Read the model definition and answer for the solid it produces. Units are mm, in the model's axes. Coordinates: 2 decimals unless noted, no trailing zeros. Order: outer loops, then holes, each group sorted by start corner. A loop starts at its lowest first (then second) coordinate and runs counter-clockwise, first axis right, second up. Notation, with made-up numbers: (42.5, 78) - (88.5, 78) arc R18 ccw to (88.5, 110) - close; hole circle Ø10 at (85, -21). An arc over 180 degrees is marked (long way). Use one line per item in the form item = value.
Autodesk Inventor part; units mm, degrees
ref_plane "YZ Plane" through (0, 0, 0) normal (1, 0, 0) x (0, 1, 0)
ref_plane "XZ Plane" through (0, 0, 0) normal (0, 1, 0) x (-1, 0, 0)
ref_plane "XY Plane" through (0, 0, 0) normal (0, 0, 1) x (1, 0, 0)
sketch "Sketch1" plane through (0, 0, 0) normal (0, 0, 1) x (1, 0, 0)
  line L0 (0, 0) -> (457.2, 0)
  line L1 (457.2, 0) -> (457.2, 304.8)
  line L2 (457.2, 304.8) -> (0, 304.8)
  line L3 (0, 304.8) -> (0, 0)
  line L4 (0, 254) -> (457.2, 254)
  arc A0 (0.6776, 254) -> (325.1105, 153.4434) centre (178.4776, 254) ccw
  circle A1 centre (178.4776, 152.4) radius 50.8
  line L5 (394.0694, 254) -> (325.1105, 153.4434)
  dimension "d0" = 457.2
  dimension "d1" = 304.8
  dimension "d4" = 101.6
sketch "Sketch2" plane through (0, 0, 0) normal (0, 0, 1) x (1, 0, 0)
  point P0 (0, 0)
extrude "Extrusion1" add sketch "Sketch1" along normal blind 6.35
properties part number "ShooterWall"
(1) Straight lines are drawn through the part: L1, parallel to Y at x = 216.5, z = 3; L2, parallel to Y at x = 171.5, z = 5; L3, parallel to X at y = 123, z = 1.5. For each, find the intervals that lie inside material, in ascending order.
Answer list:
L1 = 0 to 118.71, 186.09 to 304.8
L2 = 0 to 102.08, 202.72 to 304.8
L3 = 0 to 137.05, 219.91 to 457.2
(2) Section B-B, the plane z = 2.75 is taken. Write down the section's boundary in (x, y).
Answer list:
outline = (0, 0) - (457.2, 0) - (457.2, 304.8) - (0, 304.8) - close; hole circle Ø101.6 at (178.48, 152.4)
(3) Section A-A, the plane y = 152.4 is taken. Write down the section's boundary in (x, z).
Answer list:
outline = (0, 0) - (127.68, 0) - (127.68, 6.35) - (0, 6.35) - close; (229.28, 0) - (457.2, 0) - (457.2, 6.35) - (229.28, 6.35) - close
